Input: dimensioned drawing with shaded views. Units: mm. Origin: part minimum x, y, z. A direction names the side the tool comes from. Coordinates: 2 decimals unless noted, no trailing zeros. Write each loop counter-clockwise with the first axis right and the second up, starting at its lowest first coordinate (ties: lowest second). Pieces come first, ordered by that corner, then holes. Notation, with made-up numbers: (51.25, 61.5) - (79.25, 61.5) arc R27 ccw to (79.25, 80.5) - close; hole circle Ø1 at (40.25, 10.25). An arc over 180 degrees is marked (long way). One line per question, with ' | ' between items.
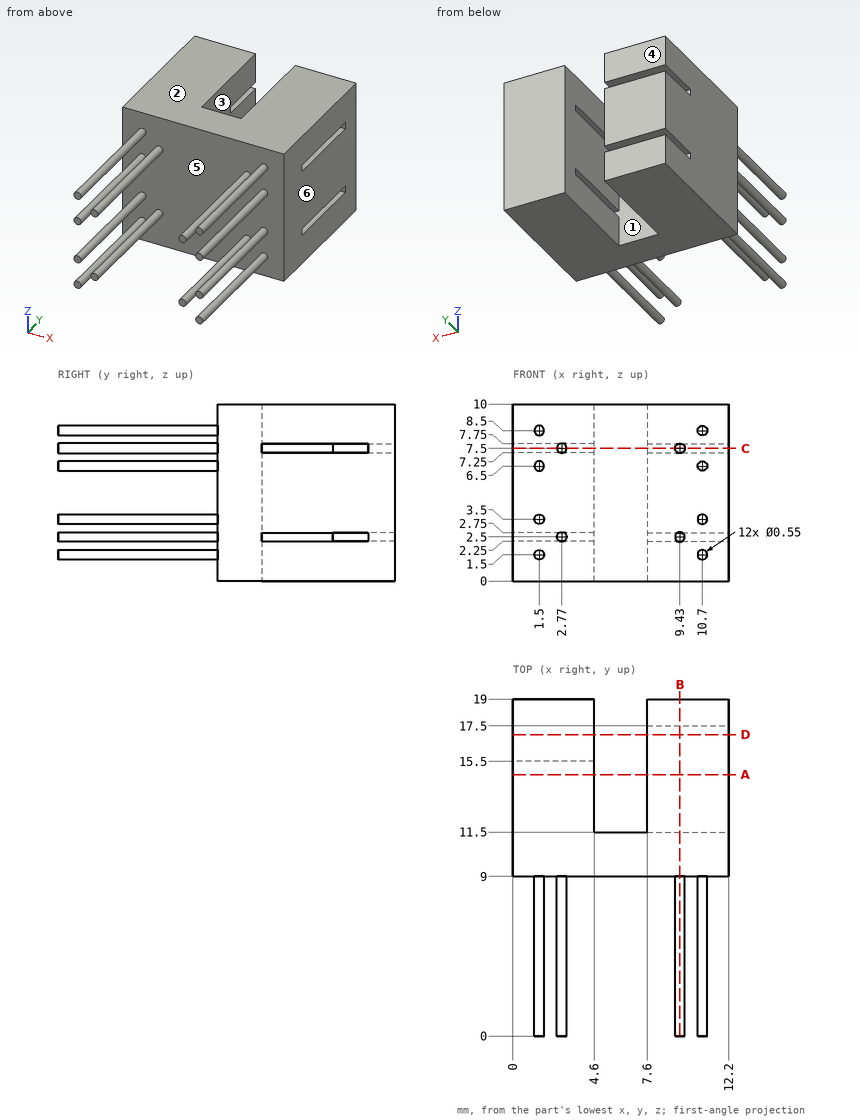
Item 1: Access query for the marked faces 1, 2 and 3. Directions: +Z, -Z, +X, -X, +Y, -Y. A direction counts if a zero-diameter tool reaches every point of the face in a straight line with its end or side. Return the directions, or none.
Check sheet entries:
face 1: none | face 2: +Z, +X, -X, +Y, -Y | face 3: +Z, -Z, +Y
Item 2: Mould query, pull axis X, two halves, no side actions, for the marked faces 4, 5 and 6. Classes: pulls with the +X half, pulls with the -X half, needs draft (parallel to the pull), parting line crosses it, or undercut.
Check sheet entries:
face 4: needs draft | face 5: undercut | face 6: pulls with the +X half
Item 3: Cut plane B-B on x = 9.43. Return loops of the section in (y, z) (3 decimals).
Check sheet entries:
outline: (0, 2.225) - (9, 2.225) - (9, 0) - (19, 0) - (19, 10) - (9, 10) - (9, 7.775) - (0, 7.775) - (0, 7.225) - (9, 7.225) - (9, 2.775) - (0, 2.775) - close; hole (11.5, 2.25) - (17.5, 2.25) - (17.5, 2.75) - (11.5, 2.75) - close; hole (11.5, 7.25) - (17.5, 7.25) - (17.5, 7.75) - (11.5, 7.75) - close
Item 4: Cut plane D-D on y = 17. Return loops of the section in (x, z).
Check sheet entries:
outline: (0, 0) - (4.6, 0) - (4.6, 2.25) - (0, 2.25) - close; (0, 2.75) - (4.6, 2.75) - (4.6, 7.25) - (0, 7.25) - close; (0, 7.75) - (4.6, 7.75) - (4.6, 10) - (0, 10) - close; (7.6, 0) - (12.2, 0) - (12.2, 2.25) - (7.6, 2.25) - close; (7.6, 2.75) - (12.2, 2.75) - (12.2, 7.25) - (7.6, 7.25) - close; (7.6, 7.75) - (12.2, 7.75) - (12.2, 10) - (7.6, 10) - close
Item 5: Cut plane A-A on y = 14.75. Return loops of the section in (x, z), and give its area (3 significant figures).
Check sheet entries:
outline: (0, 0) - (4.6, 0) - (4.6, 10) - (0, 10) - close; (7.6, 0) - (12.2, 0) - (12.2, 2.25) - (7.6, 2.25) - close; (7.6, 2.75) - (12.2, 2.75) - (12.2, 7.25) - (7.6, 7.25) - close; (7.6, 7.75) - (12.2, 7.75) - (12.2, 10) - (7.6, 10) - close | area: 87.4 mm²
Item 6: Cut plane C-C on z = 7.5. Return loops of the section in (x, y) (3 decimals), and give its area (3 significant figures).
Check sheet entries:
outline: (0, 9) - (2.495, 9) - (2.495, 0) - (3.045, 0) - (3.045, 9) - (9.155, 9) - (9.155, 0) - (9.705, 0) - (9.705, 9) - (12.2, 9) - (12.2, 11.5) - (4.6, 11.5) - (4.6, 15.5) - (0, 15.5) - close; (7.6, 17.5) - (12.2, 17.5) - (12.2, 19) - (7.6, 19) - close | area: 65.7 mm²
Item 7: Ray query, line 1 along Z through (x, y) = (10.75, 1.5); line 2 along Z through (x, y) = (10.75, 13.5); line 3 along X through (y, z) = (4.25, 2.5) (3 decimals). Return the intervals inside material, ascending. Write a range as [from, to].
Check sheet entries:
line 1: [1.23, 1.77], [3.23, 3.77], [6.23, 6.77], [8.23, 8.77] | line 2: [0, 2.25], [2.75, 7.25], [7.75, 10] | line 3: [2.495, 3.045], [9.155, 9.705]
